Design review of the part shown in the three views and the two pictorial views. Dimensions are in mm from the part's minimum x, y and z. Coordinates: 2 decimals unless noted, no trailing zeros. Loops run counter-clockwise (first coordinate to the right, second up) from the corner with the lowest first, then second, coordinate; pieces in that order, holes last. Notation, with made-up numbers: M 27.25,-26 L 50.25,-26 A28 ccw 50.25,8 Z; hole C 42,45.5 d10. An arc over 180 degrees is marked long. Answer as a JSON object with one key per item and string values. Group by question number.
Item 1: Add section C-C (y = 2.85). State the section outline as (x, z) points (1 decimal), then the cut area to 3 significant figures.
Item 2: Add section B-B (x = 55.5). State the section outline as (y, z) points.
Item 3: Mouldability with a two-part tool opening along Z and no side actions: class the marked faces 1 and 2 as +Z half, -Z half, draft (parallel to the pull), parting line (faces both ways), or undercut.
Item 4: Wall thickness on L1, parallel to Z at x = 62.5, y = 1.2; L2, parallel to Z at x = 76.5, y = 2.6 (1 decimal); L3, parallel to X at y = 0.35, z = 30 (1 decimal): over which ranges is each line inside the solid? List them lowest first. Write a range as from..to.
Item 5: Add section D-D (z = 41.5). State the section outline as (x, y) points.
Item 6: Add section A-A (z = 103.5). State the section outline as (x, y) points, then the cut area to 3 significant figures.
Item 7: Insertion check: pin 1 (1.5 mm diameter, centred on y = 2, z = 71.5, fed in from +X). The pin has a flat end and moves straight along its axis. Give the tip position at first contact, or say it passes through.
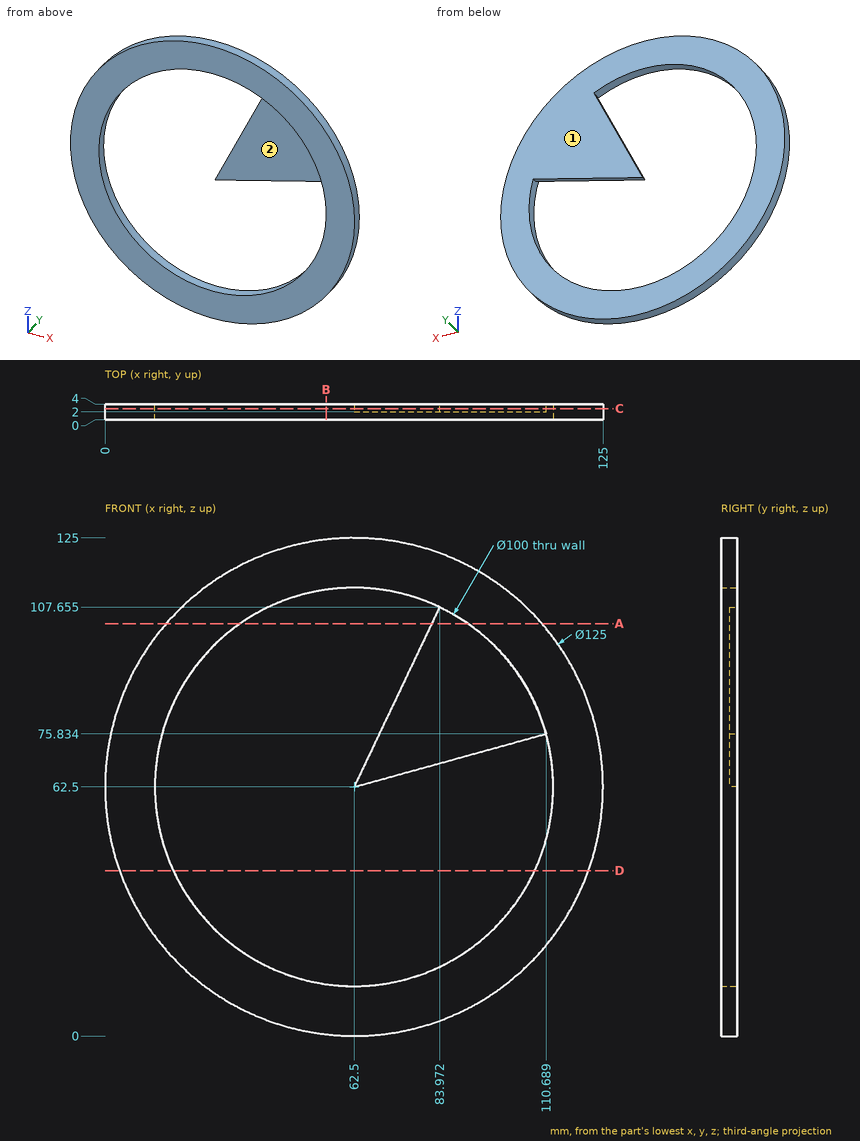
From the geometry:
{
 "1": {"outline": "C 62.5,62.5 d125; hole M 62.5,62.5 L 84,107.7 A50 ccw long 110.7,75.8 Z", "area": "5,490 mm²"},
 "2": {"outline": "M 0,0.39 L 4,0.39 L 4,12.99 L 0,12.99 Z; M 0,112.01 L 4,112.01 L 4,124.61 L 0,124.61 Z"},
 "3": {"face 1": "draft", "face 2": "undercut"},
 "4": {"L1": "z = 0..12.5, 112.5..125", "L2": "z = 1.6..14.5, 66.4..91.9, 110.5..123.4", "L3": "x = 9.1..24.5, 100.5..115.9"},
 "5": {"outline": "M 3.63,0 L 17.12,0 L 17.12,4 L 3.63,4 Z; M 107.88,0 L 121.37,0 L 121.37,4 L 107.88,4 Z"},
 "6": {"outline": "M 15.33,0 L 33.88,0 L 33.88,4 L 15.33,4 Z; M 82,2 L 91.12,2 L 91.12,0 L 109.67,0 L 109.67,4 L 82,4 Z", "area": "167 mm²"},
 "7": {"pin 1": "stops at x = 124.45"}
}
